Study the drawing (mm; zero at the part's minimum x, y, z) and answer. A direction names the side the tool comes from. Give positions to 0.01 mm unless a question says otherwise; leave off trailing zeros. Order: outer loops, then holes, each group sorted by start corner. A loop starts at its lowest first (then second) coordinate and runs counter-clockwise, first axis right, second up.
Item 1: Which of the six approach directions +Z, -Z, +X, -X, +Y, -Y give full straight-line access (tool end or side, diameter ignored) to the marked faces 1, 2 and 3?
Item 2: A cutting plane is placed at C-C (z = 9). Write down the section's boundary in (x, y).
Item 3: Given pin 1 Ø1.4 at (x, y) = (5.5, 4.5) entering from -Z; pin 2 Ø1 at (x, y) = (8, 6) entering from -Z, each flat-ended and moving along its own axis, determine where each tip first touches the part or whether it passes through.
Item 4: The mould has two halves that part along X. Classify the marked faces 4, 5 and 6: +X half, -X half, draft (parallel to the pull), parting line (faces both ways), or undercut.
Item 5: A cutting plane is placed at D-D (z = 3.75). Write down the section's boundary in (x, y), plus the area to 3 significant figures.
Item 6: A cutting plane is placed at A-A (y = 5.3). Write down the section's boundary in (x, z) (3 decimals), plus the area to 3 significant figures.
Item 7: Find the intervals of material crossed by line 1 along Y through (x, z) = (10.5, 1.5); line 2 along Y through (x, z) = (4.5, 8); line 3 along X through (y, z) = (3, 5), in increasing order.
Item 8: A cutting plane is placed at B-B (x = 6). Write down the section's boundary in (y, z).
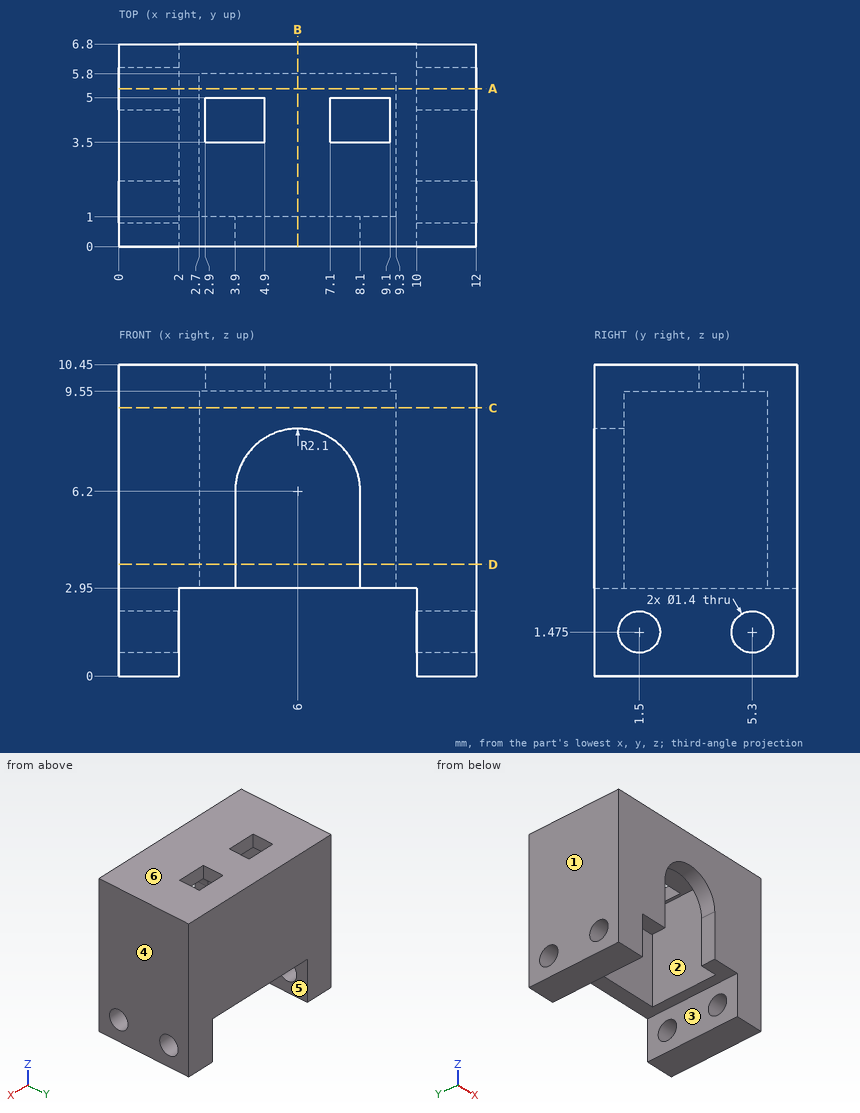
Response values:
1. face 1: +Z, -Z, -X, +Y, -Y
1. face 2: -Z
1. face 3: -Z, +Y, -Y
2. outline: (0, 0) - (12, 0) - (12, 6.8) - (0, 6.8) - close; hole (2.7, 1) - (9.3, 1) - (9.3, 5.8) - (2.7, 5.8) - close
3. pin 1: stops at z = 9.55
3. pin 2: stops at z = 2.95
4. face 4: +X half
4. face 5: undercut
4. face 6: draft
5. outline: (0, 0) - (3.9, 0) - (3.9, 1) - (2.7, 1) - (2.7, 5.8) - (9.3, 5.8) - (9.3, 1) - (8.1, 1) - (8.1, 0) - (12, 0) - (12, 6.8) - (0, 6.8) - close
5. area: 45.7 mm2
6. outline: (0, 0) - (2, 0) - (2, 0.775) - (0, 0.775) - close; (0, 2.175) - (2, 2.175) - (2, 2.95) - (2.7, 2.95) - (2.7, 9.55) - (9.3, 9.55) - (9.3, 2.95) - (10, 2.95) - (10, 2.175) - (12, 2.175) - (12, 10.45) - (0, 10.45) - close; (10, 0) - (12, 0) - (12, 0.775) - (10, 0.775) - close
6. area: 52.6 mm2
7. line 1: y = 0 to 0.8, 2.2 to 4.6, 6 to 6.8
7. line 2: y = 0 to 1, 5.8 to 6.8
7. line 3: x = 0 to 2.7, 9.3 to 12
8. outline: (0, 8.3) - (1, 8.3) - (1, 9.55) - (5.8, 9.55) - (5.8, 2.95) - (6.8, 2.95) - (6.8, 10.45) - (0, 10.45) - close
